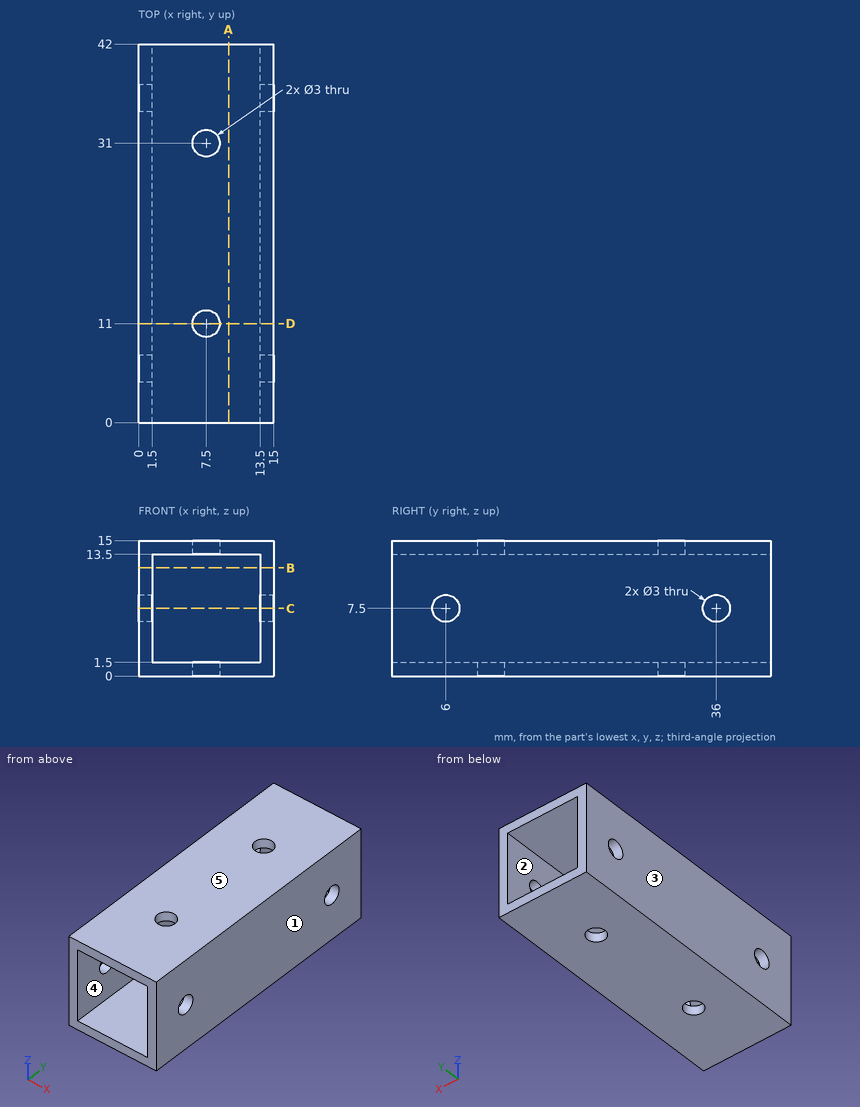
Can you work these out from the drawing? Everything is in mm from the part's minimum corner. A direction names the side the tool comes from. Round coordinates to 2 decimals unless told otherwise and drop trailing zeros. Loops run counter-clockwise (first coordinate to the right, second up) from the corner with the lowest first, then second, coordinate; pieces in that order, holes last. Notation, with made-up numbers: (46.5, 41.25) - (63.5, 41.25) arc R25 ccw to (63.5, 80.25) - close; hole circle Ø3 at (85, 6.5). An arc over 180 degrees is marked (long way). Answer in a Markdown table with one row per item. Add a question column.
(1) For the marked faces 4 and 5, which set-ups out of +Z, -Z, +X, -X, +Y, -Y let a thin tool reach every point of the face, with its end or its side?
(2) I'm going to push a flat-ended pin straight in: pin 1 (5 mm diameter, centred on y = 6, z = 7.5, fed in from +X). Where does the tip first touch, or does it pass through?
(3) If we section it at D-D (y = 11): Please give me the cut outline in (x, z), plus the area to 3 significant figures.
(4) If we mould it in two halves opening along X, with no side actions, what happens to the marked faces 1, 2 and 3? For each: pulls with the +X half, pulls with the -X half, needs draft (parallel to the pull), parting line crosses it, or undercut.
(5) If we section it at A-A (x = 10): Please give me the cut outline in (y, z), plus the area to 3 significant figures.
(6) If we section it at C-C (z = 7.5): Please give me the cut outline in (x, y), plus the area to 3 significant figures.
(7) If we section it at B-B (z = 12): Please give me the cut outline in (x, y), plus the area to 3 significant figures.
(8) I need wall thicknesses on line 1 along Y through (x, z) = (0.4, 7.5); line 2 along X through (y, z) = (15, 5.75). Which ranges of each line are inside material? Lowest first, please.
Model answer:
| question | item | result |
|---|---|---|
| 1 | face 4 | +Y, -Y |
| 1 | face 5 | +Z, +X, -X, +Y, -Y |
| 2 | pin 1 | stops at x = 15 |
| 3 | outline | (0, 0) - (6, 0) - (6, 1.5) - (1.5, 1.5) - (1.5, 13.5) - (6, 13.5) - (6, 15) - (0, 15) - close; (9, 0) - (15, 0) - (15, 15) - (9, 15) - (9, 13.5) - (13.5, 13.5) - (13.5, 1.5) - (9, 1.5) - close |
| 3 | area | 72.0 mm² |
| 4 | face 1 | pulls with the +X half |
| 4 | face 2 | undercut |
| 4 | face 3 | pulls with the -X half |
| 5 | outline | (0, 0) - (42, 0) - (42, 1.5) - (0, 1.5) - close; (0, 13.5) - (42, 13.5) - (42, 15) - (0, 15) - close |
| 5 | area | 126 mm² |
| 6 | outline | (0, 0) - (1.5, 0) - (1.5, 4.5) - (0, 4.5) - close; (0, 7.5) - (1.5, 7.5) - (1.5, 34.5) - (0, 34.5) - close; (0, 37.5) - (1.5, 37.5) - (1.5, 42) - (0, 42) - close; (13.5, 0) - (15, 0) - (15, 4.5) - (13.5, 4.5) - close; (13.5, 7.5) - (15, 7.5) - (15, 34.5) - (13.5, 34.5) - close; (13.5, 37.5) - (15, 37.5) - (15, 42) - (13.5, 42) - close |
| 6 | area | 108 mm² |
| 7 | outline | (0, 0) - (1.5, 0) - (1.5, 42) - (0, 42) - close; (13.5, 0) - (15, 0) - (15, 42) - (13.5, 42) - close |
| 7 | area | 126 mm² |
| 8 | line 1 | y = 0 to 4.5, 7.5 to 34.5, 37.5 to 42 |
| 8 | line 2 | x = 0 to 1.5, 13.5 to 15 |
